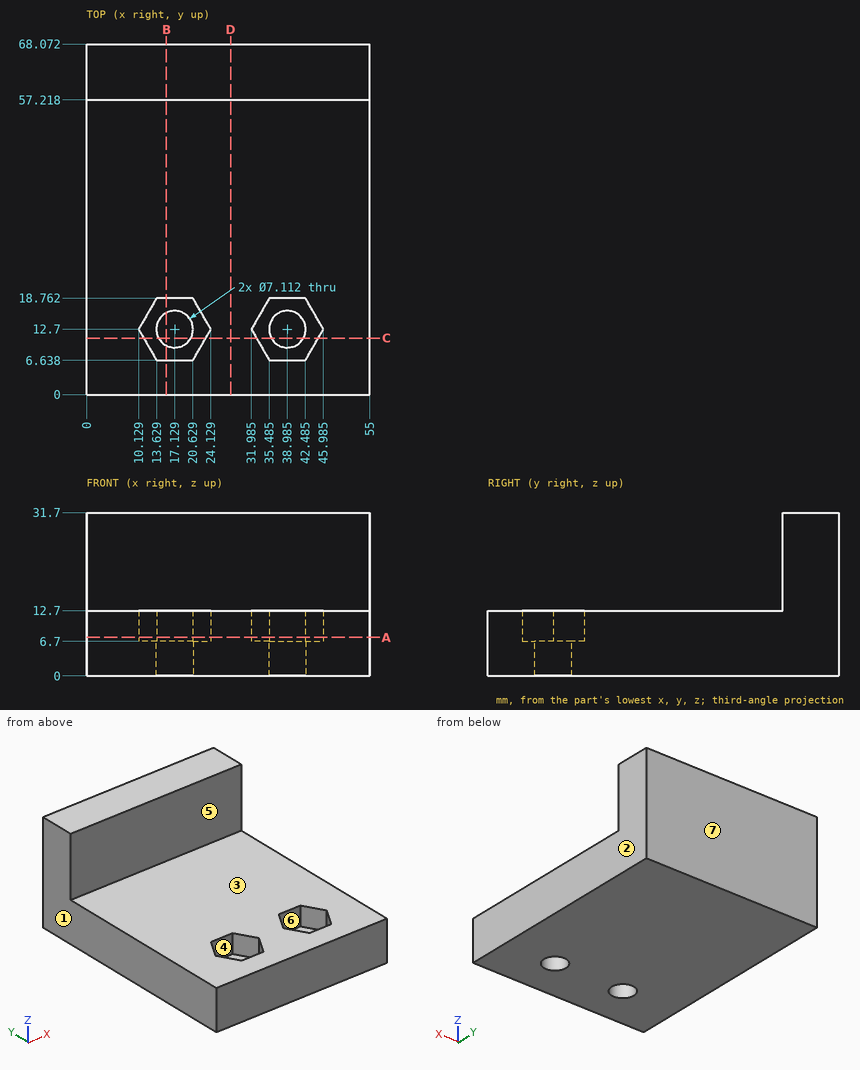
Source: three-view drawing plus pictorial views. Frame: mm from the lowest corner of the part. A direction names the side the tool comes from. Round coordinates to 2 decimals unless told otherwise and drop trailing zeros. Write each loop counter-clockwise with the first axis right and the second up, starting at its lowest first coordinate (ties: lowest second). Pieces come first, ordered by that corner, then holes. Notation, with made-up numbers: M 8.5,62.5 L 43.5,62.5 A17 ccw 43.5,93.5 Z; hole C 56,29.5 d11. An arc over 180 degrees is marked long. Use CSV: the item, a comma, the result in double quotes. Start each with the question number.
Q1. Cut plane D-D on x = 28. Output: boundary loops of the cut face in (y, z).
Q2. First-contact query: P1, Ø8, axis at x = 17.13, y = 12.7, coming from the +Z side; P2, Ø9.5, axis at x = 18, z = 17.5, coming from the -Y side; P3, Ø8, axis at x = 46.5, y = 16.5, coming from the +Z side. Flat tips, straight axial feed; report the tip coordinate or a pass-through.
Q3. Pull-direction query (X, two-part tool) for the marked faces 1, 2, 3 and 4; classes: +X half, -X half, draft (parallel to the pull), parting line (faces both ways), or undercut.
Q4. Access query for the marked faces 5, 6 and 7. Directions: +Z, -Z, +X, -X, +Y, -Y. A direction counts if a zero-diameter tool reaches every point of the face in a straight line with its end or side. Return the directions, or none.
Q5. Cut plane C-C on y = 11. Output: boundary loops of the cut face in (x, z), plus the area to 3 significant figures.
Q6. Cut plane B-B on x = 15.5. Output: boundary loops of the cut face in (y, z).
Q7. Cut plane A-A on z = 7.5. Output: boundary loops of the cut face in (x, y) (1 decimal), plus the area to 3 significant figures.
Q8. Line query: line 1 (X direction, y = 12, z = 3) (1 decimal); line 2 (Z direction, x = 42, y = 26); line 3 (Y direction, x = 48, z = 26.5). Output: solid intervals per line, ascending. Write a range as from..to.
Results found:
1,outline,"M 0,0 L 68.07,0 L 68.07,31.7 L 57.22,31.7 L 57.22,12.7 L 0,12.7 Z"
2,P1,"z = 6.7"
2,P2,"y = 57.22"
2,P3,"z = 12.7"
3,face 1,"-X half"
3,face 2,"+X half"
3,face 3,"draft"
3,face 4,"undercut"
4,face 5,"+Z, +X, -X, -Y"
4,face 6,"+Z"
4,face 7,"+Z, -Z, +X, -X, +Y"
5,outline,"M 0,0 L 14.01,0 L 14.01,6.7 L 11.11,6.7 L 11.11,12.7 L 0,12.7 Z; M 20.25,0 L 35.86,0 L 35.86,6.7 L 32.97,6.7 L 32.97,12.7 L 23.15,12.7 L 23.15,6.7 L 20.25,6.7 Z; M 42.11,0 L 55,0 L 55,12.7 L 45,12.7 L 45,6.7 L 42.11,6.7 Z"
5,area,"470 mm^2"
6,outline,"M 0,0 L 9.54,0 L 9.54,6.7 L 6.64,6.7 L 6.64,12.7 L 0,12.7 Z; M 15.86,0 L 68.07,0 L 68.07,31.7 L 57.22,31.7 L 57.22,12.7 L 18.76,12.7 L 18.76,6.7 L 15.86,6.7 Z"
7,outline,"M 0,0 L 55,0 L 55,68.1 L 0,68.1 Z; hole M 10.1,12.7 L 13.6,6.6 L 20.6,6.6 L 24.1,12.7 L 20.6,18.8 L 13.6,18.8 Z; hole M 32,12.7 L 35.5,6.6 L 42.5,6.6 L 46,12.7 L 42.5,18.8 L 35.5,18.8 Z"
7,area,"3,490 mm^2"
8,line 1,"0..13.6, 20.6..35.5, 42.5..55"
8,line 2,"0..12.7"
8,line 3,"57.22..68.07"
